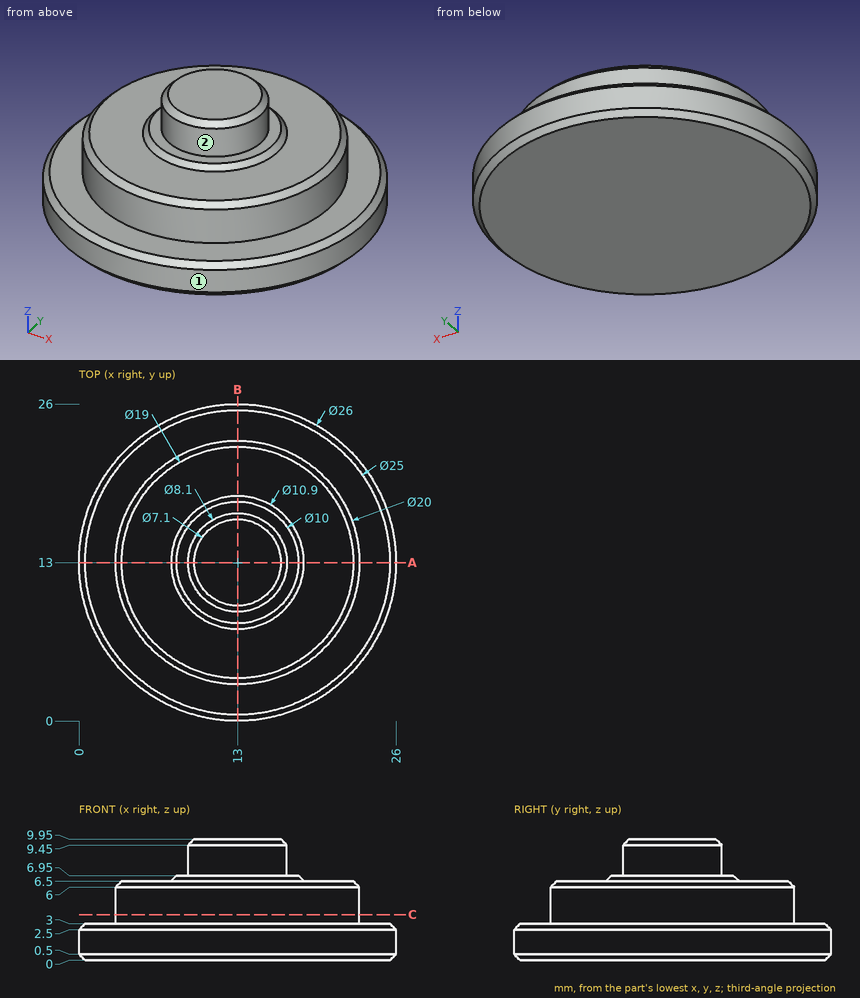
Study the drawing (mm; zero at the part's minimum x, y, z) and answer. A direction names the side the tool comes from. Coordinates: 2 decimals unless noted, no trailing zeros. Write each loop counter-clockwise with the first axis right and the second up, starting at its lowest first coordinate (ties: lowest second). Pieces come first, ordered by that corner, then holes. Notation, with made-up numbers: (-8.75, 14.25) - (33.25, 14.25) arc R8 cw to (33.25, 19.25) - close; hole circle Ø7 at (76, -9.5). An arc over 180 degrees is marked (long way). Return JSON: item names as keys, results as strings. Group by question number.
1. Straight lines are drawn through the part: L1, parallel to Z at x = 14.5, y = 7.75; L2, parallel to Z at x = 7, y = 4.25; L3, parallel to Y at x = 12.5, z = 9.75. For each, find the intervals that lie inside material, in ascending order.
2. A cutting plane is placed at C-C, the plane z = 3.75. Determine the outline of the cut face in (x, y), plus the area to 3 significant figures.
3. Which of the six approach directions +Z, -Z, +X, -X, +Y, -Y give full straight-line access (tool end or side, diameter ignored) to the marked faces 1 and 2?
4. Given pin 1 (5 mm diameter, centred on x = 20, y = 21.5, fed in from -Z); pin 2 (1.5 mm diameter, centred on y = 8.5, z = 8.5, fed in from +X); pin 3 (6 mm diameter, centred on x = 5.5, y = 21, fed in from +Z); pin 4 (3 mm diameter, centred on y = 16, z = 7, fed in from -X), each flat-ended and moving along its own axis, determine where each tip first touches the part or whether it passes through.
5. A cutting plane is placed at A-A, the plane y = 13. Determine the outline of the cut face in (x, z).
Ans:
{
 "1": {"L1": "0 to 6.5", "L2": "0 to 3", "L3": "9.28 to 16.72"},
 "2": {"outline": "circle Ø20 at (13, 13)", "area": "314 mm²"},
 "3": {"face 1": "+Z, -Z", "face 2": "+Z"},
 "4": {"pin 1": "z = 0", "pin 2": "x = 14.53", "pin 3": "z = 6.5", "pin 4": "x = 3.18"},
 "5": {"outline": "(0, 0.5) - (0.5, 0) - (25.5, 0) - (26, 0.5) - (26, 2.5) - (25.5, 3) - (23, 3) - (23, 6) - (22.5, 6.5) - (18.45, 6.5) - (18, 6.95) - (17.05, 6.95) - (17.05, 9.45) - (16.55, 9.95) - (9.45, 9.95) - (8.95, 9.45) - (8.95, 6.95) - (8, 6.95) - (7.55, 6.5) - (3.5, 6.5) - (3, 6) - (3, 3) - (0.5, 3) - (0, 2.5) - close"}
}
